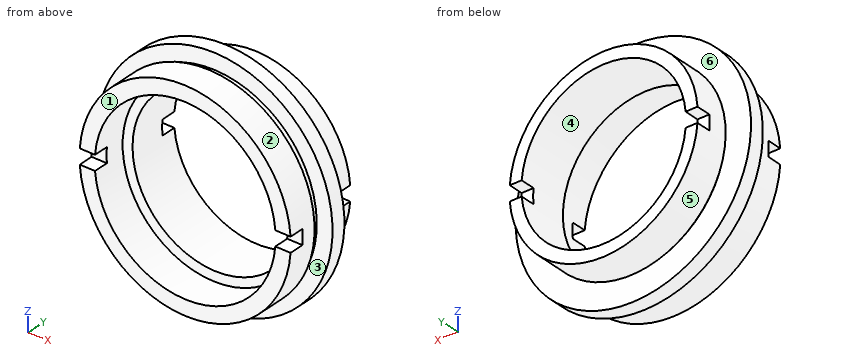
```python
from build123d import *

# Parameters (mm, degrees)
SKETCH_2_W          = 2
SKETCH_2_H          = 3.593987872
SKETCH_2_H_2        = 6.667892238
CUT_EXTRUDE_1_DEPTH = 39.5


with BuildPart() as part:
    # 草图1 → 旋转1 (revolve)
    with BuildSketch(Plane.XY, mode=Mode.PRIVATE) as revolve_1_sk:
        Polygon((-11.1, 12), (-12.7, 12), (-12.7, 7.3), (-12.4, 7.3), (-12.4, 7), (-15.875, 7), (-15.875, 5), (-13.75, 5), (-13.75, 4), (-14.25, 4), (-14.25, 0), (-12.2, 0), (-12.2, 4.7), (-12.7, 4.7), (-12.7, 5), (-11.1, 5), align=None)
    revolve(revolve_1_sk.sketch.rotate(Axis((0, 22.677499451, 0), (0, -1, 0)), 270), axis=Axis((0, 22.677499451, 0), (0, -1, 0)))  # turned: the seam where the file's is

    # 草图2 → 切除-拉伸1 (cut, symmetric)
    with BuildSketch(Plane(origin=(0, 0, 0), x_dir=(0, 0, -1), z_dir=(1, 0, 0))):
        with Locations((0, 11.796993936)):
            Rectangle(SKETCH_2_W, SKETCH_2_H)
        with Locations((0, -1.333946119)):
            Rectangle(SKETCH_2_W, SKETCH_2_H_2)
    extrude(amount=CUT_EXTRUDE_1_DEPTH, both=True, mode=Mode.SUBTRACT)


solid = part.part
```
The model under review builds one solid part; all positions refer to its coordinate system, in mm. Face numbers are marked on the shaded views. A direction names the side the tool comes from. Give positions to 0.01 mm unless a question says otherwise; leave off trailing zeros. Write each loop counter-clockwise with the first axis right and the second up, starting at its lowest first coordinate (ties: lowest second). Pieces come first, ordered by that corner, then holes. Notation, with made-up numbers: (-11, 14.25) - (-1, 14.25) arc R35 ccw to (-1, 48.25) - close; hole circle Ø8 at (65, 5). An arc over 180 degrees is marked (long way). Answer in a Markdown table with one row per item. Add a question column.
1. Tool access review of the marked faces 1, 2 and 3: name each direction out of +Z, -Z, +X, -X, +Y, -Y from which nothing blocks a thin tool from reaching the whole face with its end or side.
2. Wall thickness on line 1 along X through (y, z) = (4.8, 0); line 2 along X through (y, z) = (7.75, 0); line 3 along Y through (x, z) = (5, -10): over which ranges is each line inside the solid? List them lowest first. Write a range as [from, to].
3. We need section D-D on y = 6.25. Write out the cut boundary in (x, z) (3 decimals), then the cut area to 3 significant figures.
4. Insertion check: P1, Ø0.6, axis at x = 13, z = 0.5, coming from the -Y side; P2, Ø2, axis at x = -13.5, y = 0.5, coming from the -Z side; P3, Ø0.6, axis at x = -13, y = 1, coming from the +Z side. Each pin has a flat end and moves straight along its axis. Give the tip position at first contact, or say it passes through.
5. Draft analysis for pull direction X (two halves, no side actions). For the marked faces 4, 5 and 6, state which applies: +X half, -X half, draft (parallel to the pull), parting line (faces both ways), or undercut.
Ans:
| question | item | result |
|---|---|---|
| 1 | face 1 | +Z, -Z, +X, -X, -Y |
| 1 | face 2 | -Y |
| 1 | face 3 | none |
| 2 | line 1 | x = [-13.75, -12.7], [12.7, 13.75] |
| 2 | line 2 | x = [-12.7, -11.1], [11.1, 12.7] |
| 2 | line 3 | y = [5, 12] |
| 3 | outline | circle Ø31.75 at (0, 0); hole circle Ø22.2 at (0, 0) |
| 3 | area | 405 mm^2 |
| 4 | P1 | stops at y = 2 |
| 4 | P2 | stops at z = -6.84 |
| 4 | P3 | stops at z = 6.46 |
| 5 | face 4 | undercut |
| 5 | face 5 | parting line |
| 5 | face 6 | draft |
